Autodesk Inventor part; units mm, degrees
ref_plane "作業平面1" through (0, 0, 4.5) normal (0, 0, 1) x (1, 0, 0)
ref_plane "YZ Plane" through (0, 0, 0) normal (1, 0, 0) x (0, 1, 0)
ref_plane "XZ Plane" through (0, 0, 0) normal (0, 1, 0) x (-1, 0, 0)
sketch "スケッチ1" plane through (0, 0, 0) normal (0, 0, 1) x (1, 0, 0)
  circle A0 centre (0, 0) radius 1.6
  circle A1 centre (0, 0) radius 3
  dimension "d0" = 3.2
  dimension "d1" = 6
extrude "押し出し1" add sketch "スケッチ1" along normal blind 2.5
sketch "スケッチ2" plane through (0, 0, 0) normal (1, 0, 0) x (0, 1, 0)
  arc A0 (2.85, 3.5) -> (-2.85, 3.5) centre (0, -0.0613) ccw
  line L0 (2.85, 3.5) -> (-2.85, 3.5)
  line L1 (-2.85, 3.5) -> (-2.85, 2.5)
  line L2 (-2.85, 2.5) -> (2.85, 2.5)
  line L3 (2.85, 2.5) -> (2.85, 3.5)
  line L4 (3, 2.5) -> (-3, 2.5)
  line L5 (10, 4.5) -> (-10, 4.5)
  line L6 (0, 2.5) -> (0, 4.5)
  point P0 (0, 0)
  point P1 (0, 4.5)
  dimension "d4" = 1
  dimension "d5" = 1
  dimension "d7" = 5.7
revolve "回転1" add sketch "スケッチ2" angle 360 about axis through (0, 0, 2.5) along (0, 0, 1) picked at (1.6112, 3.682) contours L0 L6 A0 | L3 L2 L6 L0
ref_plane "作業平面1" through (0, 0, 4.5) normal (0, 0, 1) x (1, 0, 0)
sketch "スケッチ3" plane through (0, 0, 4.5) normal (0, 0, 1) x (1, 0, 0)
  line L0 (2.25, -0.5) -> (-2.25, -0.5)
  line L1 (-2.25, -0.5) -> (-2.25, 0.5)
  line L2 (-2.25, 0.5) -> (2.25, 0.5)
  line L3 (2.25, 0.5) -> (2.25, -0.5)
  line L4 (2.25, -0.5) -> (-2.25, 0.5) construction
  line L5 (-2.25, -0.5) -> (2.25, 0.5) construction
  line L6 (-0.5, -2.25) -> (0.5, -2.25)
  line L7 (0.5, -2.25) -> (0.5, 2.25)
  line L8 (0.5, 2.25) -> (-0.5, 2.25)
  line L9 (-0.5, 2.25) -> (-0.5, -2.25)
  line L10 (-0.5, -2.25) -> (0.5, 2.25) construction
  line L11 (0.5, -2.25) -> (-0.5, 2.25) construction
  point P0 (0, 0)
  point P1 (-0.5, 0.5)
  point P2 (-0.5, -0.5)
  point P3 (0.5, -0.5)
  point P4 (0.5, 0.5)
  dimension "d9" = 4.5
  dimension "d10" = 1
extrude "押し出し2" cut sketch "スケッチ3" against normal blind 1
sketch "スケッチ4" plane through (0, 0, 0) normal (0, 0, -1) x (-1, 0, 0)
  circle A0 centre (0, 0) radius 3
extrude "押し出し3" cut sketch "スケッチ4" against normal up to surface (2.5 mm away)
properties part number "screw_M3" material "アルミニウム 6061"
Here's how the part is built. I have some questions about the finished solid (model axes, mm). Give positions to 0.01 mm unless a question says otherwise; leave off trailing zeros. Order: outer loops, then holes, each group sorted by start corner. A loop starts at its lowest first (then second) coordinate and runs counter-clockwise, first axis right, second up. Notation, with made-up numbers: M -20,-12.75 L -1,-12.75 A35 ccw -1,26.25 Z; hole C 26.25,-9 d9. An arc over 180 degrees is marked long. Use a Markdown table: item, result. Add a question column.
1. Suppose I cut it at A-A (x = 0). List the corners of the cut face in (y, z) for me, and give its area (3 significant figures).
2. Suppose I cut it at D-D (z = 3.25). List the corners of the cut face in (x, y) for me.
3. If we mould it in two halves opening along X, with no side actions, what happens to faces 1 (the flat face through (0.5, -1, 4)), 2 (the cylindrical face through (1.734, -2.262, 3.007)), 3 (the flat face through (0, 0, 2.5))? For each: +X half, -X half, draft (parallel to the pull), parting line (faces both ways), or undercut.
4. Suppose I cut it at C-C (z = 3.65). List the corners of the cut face in (x, y) for me, and give its area (3 significant figures).
5. I need wall thicknesses on probe 1 along Z at (x, y) = (-0.4, -1); probe 2 along X at (y, z) = (1.55, 3.9); probe 3 along Y at (x, z) = (-0.8, 2.7). Which ranges of each line are inside material? Lowest first, please. Write a range as from..to.
6. For pin 1 Ø0.8 at (y, z) = (-1.5, 4) entering from -X; pin 2 Ø0.8 at (y, z) = (-1, 4) entering from +X; pin 3 Ø1 at (x, z) = (-1, 4) entering from -Y, each with a flat end and sliding along its axis, tell me the tip position at first contact or that it passes through.
7. Suppose I cut it at B-B (y = 1.2). List the corners of the cut face in (x, z) for me.
Results list:
| question | item | result |
|---|---|---|
| 1 | outline | M -2.85,2.5 L 2.85,2.5 L 2.85,3.5 A4.56 ccw 2.25,3.91 L 2.25,3.5 L -2.25,3.5 L -2.25,3.91 A4.56 ccw -2.85,3.5 Z |
| 1 | area | 5.96 mm² |
| 2 | outline | C 0,0 d5.7 |
| 3 | face 1 | undercut |
| 3 | face 2 | parting line |
| 3 | face 3 | draft |
| 4 | outline | C 0,0 d5.3; hole M -2.25,-0.5 L -0.5,-0.5 L -0.5,-2.25 L 0.5,-2.25 L 0.5,-0.5 L 2.25,-0.5 L 2.25,0.5 L 0.5,0.5 L 0.5,2.25 L -0.5,2.25 L -0.5,0.5 L -2.25,0.5 Z |
| 4 | area | 14.1 mm² |
| 5 | probe 1 | z = 2.5..3.5 |
| 5 | probe 2 | x = -1.65..-0.5, 0.5..1.65 |
| 5 | probe 3 | y = -2.74..2.74 |
| 6 | pin 1 | stops at x = -2.32 |
| 6 | pin 2 | stops at x = 2.55 |
| 6 | pin 3 | stops at y = -2.69 |
| 7 | outline | M -2.59,2.5 L 2.59,2.5 L 2.59,3.5 A4.4 ccw 0.5,4.31 L 0.5,3.5 L -0.5,3.5 L -0.5,4.31 A4.4 ccw -2.59,3.5 Z |
